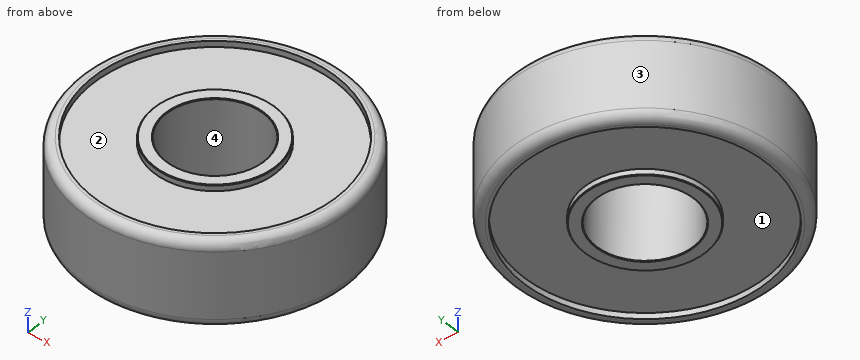
from build123d import *

# Parameters (mm, degrees)
ESQUISSE1_R             = 11
ESQUISSE1_R_2           = 4
BOSS_EXTRU_1_DEPTH      = 7
ESQUISSE2_R             = 10
ESQUISSE2_R_2           = 5
ENL_V_MAT_EXTRU_1_DEPTH = 0.5
ENL_V_START             = -0.5
ESQUISSE3_R             = 10
ESQUISSE3_R_2           = 5
ENL_V_MAT_EXTRU_2_DEPTH = 0.5
CONG_1_R                = 0.75
CHANFREIN1_SIZE         = 0.05


with BuildPart() as part:
    # Esquisse1 → Boss.-Extru.1 (new body)
    with BuildSketch(Plane.XY):
        Circle(ESQUISSE1_R)
        Circle(ESQUISSE1_R_2, mode=Mode.SUBTRACT)
    extrude(amount=BOSS_EXTRU_1_DEPTH)

    # Esquisse2 → Enlèv. mat.-Extru.1 (cut)
    with BuildSketch(Plane.XY.offset(7)):
        Circle(ESQUISSE2_R)
        Circle(ESQUISSE2_R_2, mode=Mode.SUBTRACT)
    extrude(amount=-ENL_V_MAT_EXTRU_1_DEPTH, mode=Mode.SUBTRACT)

    # Esquisse3 → Enlèv. mat.-Extru.2 (cut)
    with BuildSketch(Plane(origin=(0, 0, 0), x_dir=(-1, 0, 0), z_dir=(0, 0, -1)).offset(ENL_V_START)):
        with Locations(Location((0, 0, 0), (0, 0, 180))):
            Circle(ESQUISSE3_R)
        with Locations(Location((0, 0, 0), (0, 0, 180))):
            Circle(ESQUISSE3_R_2, mode=Mode.SUBTRACT)
    extrude(amount=ENL_V_MAT_EXTRU_2_DEPTH, mode=Mode.SUBTRACT)

    # Congé1
    cong_1_edges = [part.edges().sort_by_distance(p)[0] for p in [
        (-11, 0, 0),
        (-11, 0, 7),
    ]]
    fillet(cong_1_edges, radius=CONG_1_R)

    # Chanfrein1
    chanfrein1_edges = [part.edges().sort_by_distance(p)[0] for p in [
        (-5, 0, 7),
        (-5, 0, 0),
        (-4, 0, 0),
        (-4, 0, 7),
    ]]
    chamfer(chanfrein1_edges, length=CHANFREIN1_SIZE)


solid = part.part
Can you work these out from the model? Positions are in its coordinate system, mm. Face numbers are marked on the shaded views. A direction names the side the tool comes from. Round coordinates to 2 decimals unless told otherwise and drop trailing zeros. Write each loop counter-clockwise with the first axis right and the second up, starting at its lowest first coordinate (ties: lowest second). Pieces come first, ordered by that corner, then holes. Notation, with made-up numbers: M 70,41 L 99,41 A29 ccw 99,67 Z; hole C 18,17.25 d4. An arc over 180 degrees is marked long. Use a Markdown table: item, result.
Item 1: We'd pull the mould along X, two halves only. Please class the marked faces 3 and 4: released by +X, released by -X, zero draft, split by the parting line, or undercut.
Found:
| item | result |
|---|---|
| face 3 | split by the parting line |
| face 4 | undercut |
Item 2: Which directions (+Z, -Z, +X, -X, +Y, -Y) give clear straight access to the entire face, cutting with the end or side of a thin tool? Please do the marked faces 1 and 2.
Found:
| item | result |
|---|---|
| face 1 | -Z |
| face 2 | +Z |
Item 3: I want a section at A-A (z = 4.5). List the corners of the cut face in (x, y) for me, and give its area (3 significant figures).
Found:
| item | result |
|---|---|
| outline | C 0,0 d22; hole C 0,0 d8 |
| area | 330 mm2 |
Item 4: For pin 1 Ø2 at (y, z) = (6.5, 2) entering from +X; pin 2 Ø7 at (x, y) = (0, 0) entering from +Z; pin 3 Ø4 at (y, z) = (-5.5, 2.5) entering from -X, each with a flat end and sliding along its axis, tell me the tip position at first contact or that it passes through.
Found:
| item | result |
|---|---|
| pin 1 | stops at x = 9.53 |
| pin 2 | passes through |
| pin 3 | stops at x = -10.43 |
Item 5: If I drill on line 1 along Y through (x, z) = (0, 0.25); line 2 along Y through (x, z) = (0, 5); line 3 along Y through (x, z) = (0, 6.6), over which ranges is the centre line in solid material (lowest first)? Write a range as [from, to].
Found:
| item | result |
|---|---|
| line 1 | y = [-10.81, -10], [-5, -4], [4, 5], [10, 10.81] |
| line 2 | y = [-11, -4], [4, 11] |
| line 3 | y = [-10.91, -10], [-5, -4], [4, 5], [10, 10.91] |
